Here's the drawing with two shaded views (mm, measured from the low corner). I have some questions. A direction names the side the tool comes from. Give positions to 0.01 mm unless a question says otherwise; leave off trailing zeros. Write each loop counter-clockwise with the first axis right and the second up, starting at its lowest first coordinate (ties: lowest second). Pieces come first, ordered by that corner, then holes.
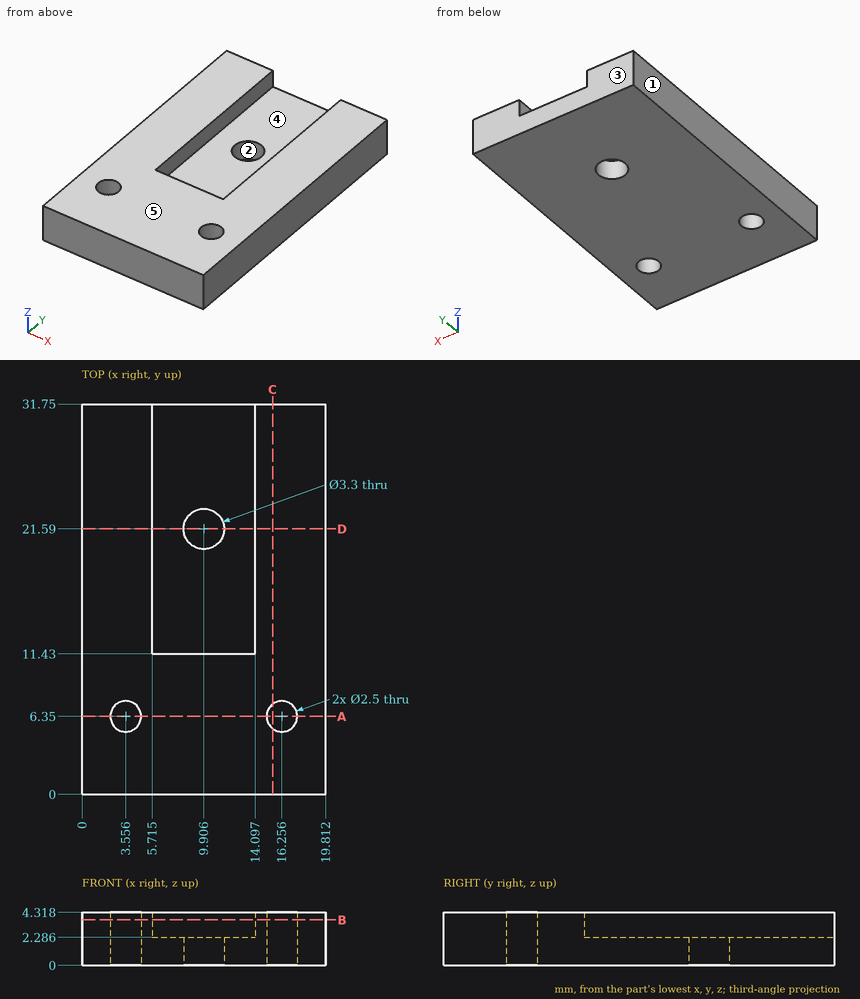
1) Suppose I cut it at B-B on z = 3.7. Write out the boundary of the cut face in (x, y) (3 decimals), plus the area to 3 significant figures.
Values follow:
outline: (0, 0) - (19.812, 0) - (19.812, 31.75) - (14.097, 31.75) - (14.097, 11.43) - (5.715, 11.43) - (5.715, 31.75) - (0, 31.75) - close; hole circle Ø2.5 at (3.556, 6.35); hole circle Ø2.5 at (16.256, 6.35)
area: 449 mm2
2) Please list where these lines run through material, in increasing order: L1, parallel to X at y = 23, z = 2.55 (3 decimals); L2, parallel to Y at x = 3.5, z = 1.3; L3, parallel to Y at x = 9.75, z = 0.6.
Values follow:
L1: x = 0 to 5.715, 14.097 to 19.812
L2: y = 0 to 5.1, 7.6 to 31.75
L3: y = 0 to 19.95, 23.23 to 31.75
3) For pin 1 Ø1 at (x, z) = (9, 3.5) entering from +Y; pin 2 Ø4 at (x, y) = (11, 28) entering from +Z, each with a flat end and sliding along its axis, tell me the tip position at first contact or that it passes through.
Values follow:
pin 1: stops at y = 11.43
pin 2: stops at z = 2.29
4) For the marked faces 4 and 5, which set-ups out of +Z, -Z, +X, -X, +Y, -Y let a thin tool reach every point of the face, with its end or its side?
Values follow:
face 4: +Z, +Y
face 5: +Z, +X, -X, +Y, -Y
5) If we mould it in two halves opening along X, with no side actions, what happens to the marked faces 1, 2 and 3? For each: +X half, -X half, draft (parallel to the pull), parting line (faces both ways), or undercut.
Values follow:
face 1: -X half
face 2: undercut
face 3: draft
6) Suppose I cut it at A-A on y = 6.35. Write out the boundary of the cut face in (x, z).
Values follow:
outline: (0, 0) - (2.31, 0) - (2.31, 4.32) - (0, 4.32) - close; (4.81, 0) - (15.01, 0) - (15.01, 4.32) - (4.81, 4.32) - close; (17.51, 0) - (19.81, 0) - (19.81, 4.32) - (17.51, 4.32) - close
7) Suppose I cut it at C-C on x = 15.5. Write out the boundary of the cut face in (y, z).
Values follow:
outline: (0, 0) - (5.35, 0) - (5.35, 4.32) - (0, 4.32) - close; (7.35, 0) - (31.75, 0) - (31.75, 4.32) - (7.35, 4.32) - close
8) Suppose I cut it at D-D on y = 21.59. Write out the boundary of the cut face in (x, z) (3 decimals).
Values follow:
outline: (0, 0) - (8.256, 0) - (8.256, 2.286) - (5.715, 2.286) - (5.715, 4.318) - (0, 4.318) - close; (11.556, 0) - (19.812, 0) - (19.812, 4.318) - (14.097, 4.318) - (14.097, 2.286) - (11.556, 2.286) - close
